from build123d import *

# Parameters (mm, degrees)
F0_R     = 9.525
F1_DEPTH = 127
F2_W     = 228.6
F2_H     = 152.4
F3_DEPTH = 113.538


with BuildPart() as f1:
    # F0 (on Right) → F1 (new body, symmetric)
    with BuildSketch(Plane.YZ):
        with BuildLine():
            ThreePointArc((-11.821697, 4.640849), (-2.361614, -12.478493), (12.7, 0))
            ThreePointArc((12.7, 0), (12.478493, 2.361614), (11.821697, 4.640849))
            ThreePointArc((11.821697, 4.640849), (0, 12.7), (-11.821697, 4.640849))
        make_face()
        Circle(F0_R, mode=Mode.SUBTRACT)
        with BuildLine():
            ThreePointArc((11.821697, 4.640849), (12.478493, 2.361614), (12.7, 0))
            ThreePointArc((12.7, 0), (-2.361614, -12.478493), (-11.821697, 4.640849))
            Line((-11.821697, 4.640849), (-63.5, -127))
            Line((-63.5, -127), (63.5, -127))
            Line((63.5, -127), (11.821697, 4.640849))
        make_face()
    extrude(amount=F1_DEPTH, both=True)

    # F2 (on Front) → F3 (cut, symmetric)
    with BuildSketch(Plane.XZ):
        with Locations((0, -38.1)):
            Rectangle(F2_W, F2_H)
    extrude(amount=F3_DEPTH, both=True, mode=Mode.SUBTRACT)


solid = f1.part
Verification items for the finished model (mm, model axes). A direction names the side the tool comes from. Round coordinates to 2 decimals unless told otherwise and drop trailing zeros. Loops run counter-clockwise (first coordinate to the right, second up) from the corner with the lowest first, then second, coordinate; pieces in that order, holes last. Notation, with made-up numbers: (8, 51) - (41, 51) arc R15 ccw to (41, 60) - close; hole circle Ø4 at (31.5, -13.5). An arc over 180 degrees is marked (long way). Write item = value, one per line.
Q1. Sectioned sample at B-B on z = -79. Record the boundary of the cut face in (x, y), plus the area to 3 significant figures.
Here are the results:
outline = (-127, -44.66) - (-114.3, -44.66) - (-114.3, 44.66) - (-127, 44.66) - close; (114.3, -44.66) - (127, -44.66) - (127, 44.66) - (114.3, 44.66) - close
area = 2,270 mm^2
Q2. Sectioned sample at C-C on z = 0. Record the boundary of the cut face in (x, y) (3 decimals), plus the area to 3 significant figures.
Here are the results:
outline = (-127, -13.644) - (-114.3, -13.644) - (-114.3, -9.525) - (-127, -9.525) - close; (-127, 9.525) - (-114.3, 9.525) - (-114.3, 13.644) - (-127, 13.644) - close; (114.3, -13.644) - (127, -13.644) - (127, -9.525) - (114.3, -9.525) - close; (114.3, 9.525) - (127, 9.525) - (127, 13.644) - (114.3, 13.644) - close
area = 209 mm^2
Q3. Material ranges on L1, parallel to X at y = 28, z = -85; L2, parallel to Z at x = 120.5, y = 0 (3 decimals); L3, parallel to Z at x = -53, y = 1, recorded low to high.
Here are the results:
L1 = -127 to -114.3, 114.3 to 127
L2 = -127 to -9.525, 9.525 to 12.7
L3 = -127 to -114.3
Q4. Sectioned sample at D-D on y = -19.5. Record the boundary of the cut face in (x, z).
Here are the results:
outline = (-127, -127) - (127, -127) - (127, -14.92) - (114.3, -14.92) - (114.3, -114.3) - (-114.3, -114.3) - (-114.3, -14.92) - (-127, -14.92) - close
Q5. Depth check by flat-ended pin: pin 1 (1.5 mm diameter, centred on y = -18.5, z = -7.5, fed in from +X); pin 2 (25 mm diameter, centred on y = 0, z = 0, fed in from -X); pin 3 (12 mm diameter, centred on x = -93, y = 16.5, fed in from +Z). Enter the tip coordinate at first touch or a pass-through.
Here are the results:
pin_1 = through
pin_2 = -127
pin_3 = -114.3
Q6. Tool access check on faces 1 (the flat face through (-127, -1, -72)), 2 (the flat face through (114.3, -1, -66)). Record the directions out of +Z, -Z, +X, -X, +Y, -Y that give a thin tool (end or side, any length) a straight path to the whole face; none if there is none.
Here are the results:
face_1 = +Z, -Z, -X, +Y, -Y
face_2 = +Z, +Y, -Y
Q7. Mould release check, pull along X, two halves, no side actions. Record for faces 3 (the flat face through (2, -1, -127)), 4 (the flat face through (-114.3, -1, -66)), 5 (the flat face through (127, -1, -72)): +X half, -X half, draft (parallel to the pull), parting line (faces both ways), or undercut.
Here are the results:
face_3 = draft
face_4 = undercut
face_5 = +X half
Q8. Sectioned sample at A-A on y = 0. Record the boundary of the cut face in (x, z) (3 decimals).
Here are the results:
outline = (-127, -127) - (127, -127) - (127, -9.525) - (114.3, -9.525) - (114.3, -114.3) - (-114.3, -114.3) - (-114.3, -9.525) - (-127, -9.525) - close; (-127, 9.525) - (-114.3, 9.525) - (-114.3, 12.7) - (-127, 12.7) - close; (114.3, 9.525) - (127, 9.525) - (127, 12.7) - (114.3, 12.7) - close
